Source: CAD feature listing. Evaluate the final solid. Frame: model axes, mm. Face numbers are marked on the shaded views. A direction names the side the tool comes from. Round coordinates to 2 decimals unless told otherwise and drop trailing zeros. Loops run counter-clockwise (first coordinate to the right, second up) from the corner with the lowest first, then second, coordinate; pieces in that order, holes last. Notation, with made-up numbers: (0.25, 18) - (48.25, 18) arc R30 cw to (48.25, 43) - close; hole circle Ø7 at (-17.5, 62.5). An arc over 180 degrees is marked (long way). Write item = value, one per line. Start each with the question number.
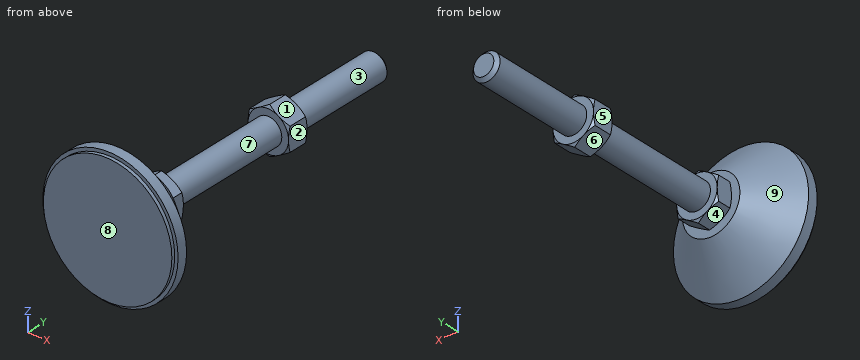
from build123d import *

# Parameters (mm, degrees)
EXTRUDE_1_DEPTH = 10
EXTRUDE_2_DEPTH = 13


with BuildPart() as part:
    # Эскиз1 → Повернуть1 (revolve)
    with BuildSketch(Plane.XY, mode=Mode.PRIVATE) as revolve_1_sk:
        Polygon((0, 0), (-38, 0), (-38, 2), (-40, 2), (-40, 8), (-17, 29), (-8, 29), (-8, 39), (-8, 187), (-6, 189), (0, 189), align=None)
    revolve(revolve_1_sk.sketch.rotate(Axis((0, 0, 0), (0, 1, 0)), 180), axis=Axis((0, 0, 0), (0, 1, 0)))  # turned: the seam where the file's is

    # Эскиз2 → Бобышка-Вытянуть1 (add)
    with BuildSketch(Plane(origin=(0, 29, 0), x_dir=(1, 0, 0), z_dir=(0, 1, 0))):
        Polygon((0, 13.856406461), (-12, 6.92820323), (-12, -6.92820323), (0, -13.856406461), (12, -6.92820323), (12, 6.92820323), align=None)
    extrude(amount=EXTRUDE_1_DEPTH)

    # Эскиз3 → Бобышка-Вытянуть2 (add)
    with BuildSketch(Plane(origin=(0, 113, 0), x_dir=(1, 0, 0), z_dir=(0, 1, 0))):
        Polygon((12, 6.92820323), (0, 13.856406461), (-12, 6.92820323), (-12, -6.92820323), (0, -13.856406461), (12, -6.92820323), align=None)
    extrude(amount=EXTRUDE_2_DEPTH)

    # Эскиз4 → Вырез-Повернуть2 (revolve, cut)
    with BuildSketch(Plane.XY, mode=Mode.PRIVATE) as cut_revolve_2_sk:
        Polygon((-23.258330249, 126), (-12, 126), (-23.258330249, 119.5), align=None)
        Polygon((-23.258330249, 113), (-23.258330249, 119.5), (-12, 113), align=None)
        Polygon((-20.660254038, 39), (-20.660254038, 34), (-12, 39), align=None)
        Polygon((-20.660254038, 34), (-20.660254038, 29), (-12, 29), align=None)
    revolve(cut_revolve_2_sk.sketch.rotate(Axis((0, 189, 0), (0, -1, 0)), 180), axis=Axis((0, 189, 0), (0, -1, 0)), mode=Mode.SUBTRACT)  # turned: the seam where the file's is


solid = part.part
(1) Mould query, pull axis Y, two halves, no side actions, for the marked faces 6, 7, 8 and 9. Classes: +Y half, -Y half, draft (parallel to the pull), parting line (faces both ways), or undercut.
(2) Pin query (flat end, axial travel): P1, Ø19, axis at x = -3, z = 5, coming from the -Y side; P2, Ø11, axis at y = 34, z = -0.5, coming from the -X side; P3, Ø3, axis at y = 143, z = 10.5, coming from the -X side; P4, Ø6.5, axis at y = 122.5, z = 1.5, coming from the +X side. Return the tip coordinate at first contact, or that it passes through.
(3) Cut plane A-A (y = 167). Output: boundary loops of the cut face in (x, z).
(4) Material intervals for line 1 along Y through (x, z) = (-2, -10.5); line 2 along Y through (x, z) = (28, -22); line 3 along Y through (x, z) = (-17, 29), sorted ascending. Write a range as from..to.
(5) Access query for the marked faces 1, 2, 3, 4 and 5. Directions: +Z, -Z, +X, -X, +Y, -Y. A direction counts if a zero-diameter tool reaches every point of the face in a straight line with its end or side. Return the directions, or none.
Solution:
q1.face_6 = draft
q1.face_7 = undercut
q1.face_8 = -Y half
q1.face_9 = +Y half
q2.P1 = 0
q2.P2 = -17.54
q2.P3 = through
q2.P4 = 12
q3.outline = circle Ø16 at (0, 0)
q4.line_1 = 0..39, 113..126
q4.line_2 = 0..12.01
q4.line_3 = 0..13.83
q5.face_1 = +Z, +X, +Y
q5.face_2 = +Z, -Z, +X, +Y
q5.face_3 = +Y
q5.face_4 = -Z, -X, +Y
q5.face_5 = +Z, -Z, -X, +Y
